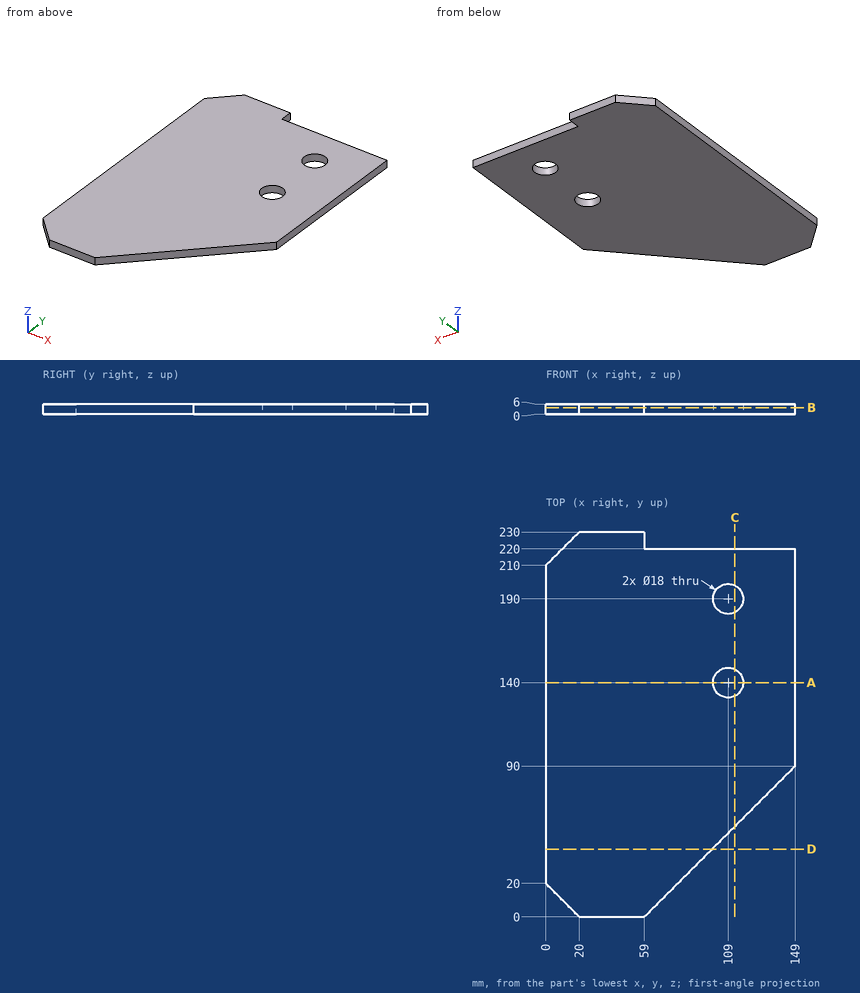
The drawing under review shows one solid part. Ordinate dimensions are in mm from its lowest x, y, z. Round coordinates to 2 decimals unless told otherwise and drop trailing zeros. Write each loop counter-clockwise with the first axis right and the second up, starting at its lowest first coordinate (ties: lowest second). Pieces come first, ordered by that corner, then holes. Notation, with made-up numbers: (34, 66) - (82, 66) arc R19 ccw to (82, 84) - close; hole circle Ø8 at (41.5, 49). An arc over 180 degrees is marked (long way). Use one line per item in the form item = value.
Q1. Consider section A-A (y = 140). State the section outline as (x, z) points, and give its area (3 significant figures).
Answer key:
outline = (0, 0) - (100, 0) - (100, 6) - (0, 6) - close; (118, 0) - (149, 0) - (149, 6) - (118, 6) - close
area = 786 mm2
Q2. Consider section B-B (z = 3.9). State the section outline as (x, y) points.
Answer key:
outline = (0, 20) - (20, 0) - (59, 0) - (149, 90) - (149, 220) - (59, 220) - (59, 230) - (20, 230) - (0, 210) - close; hole circle Ø18 at (109, 140); hole circle Ø18 at (109, 190)
Q3. For line 1 (X direction, y = 140, z = 1.5); line 2 (Y direction, x = 109, z = 4.5); line 3 (X direction, y = 136.5, z = 4.5), list the stretches that pass through material, from the lowest coordinate up. Write a range as [from, to].
Answer key:
line_1 = [0, 100], [118, 149]
line_2 = [50, 131], [149, 181], [199, 220]
line_3 = [0, 100.71], [117.29, 149]
Q4. Consider section D-D (y = 40.5). State the section outline as (x, z) points, and give its area (3 significant figures).
Answer key:
outline = (0, 0) - (99.5, 0) - (99.5, 6) - (0, 6) - close
area = 597 mm2
Q5. Insertion check: pin 1 Ø3 at (x, z) = (91.5, 2.5) entering from -Y; pin 2 Ø1 at (x, z) = (112.5, 2.5) entering from -Y; pin 3 Ø1.8 at (y, z) = (224, 3.5) entering from +X. Each pin has a flat end and moves straight along its axis. Give the tip position at first contact, or say it passes through.
Answer key:
pin_1 = 31
pin_2 = 53
pin_3 = 59
Q6. Consider section C-C (x = 113). State the section outline as (y, z) points, and give its area (3 significant figures).
Answer key:
outline = (54, 0) - (131.94, 0) - (131.94, 6) - (54, 6) - close; (148.06, 0) - (181.94, 0) - (181.94, 6) - (148.06, 6) - close; (198.06, 0) - (220, 0) - (220, 6) - (198.06, 6) - close
area = 803 mm2
